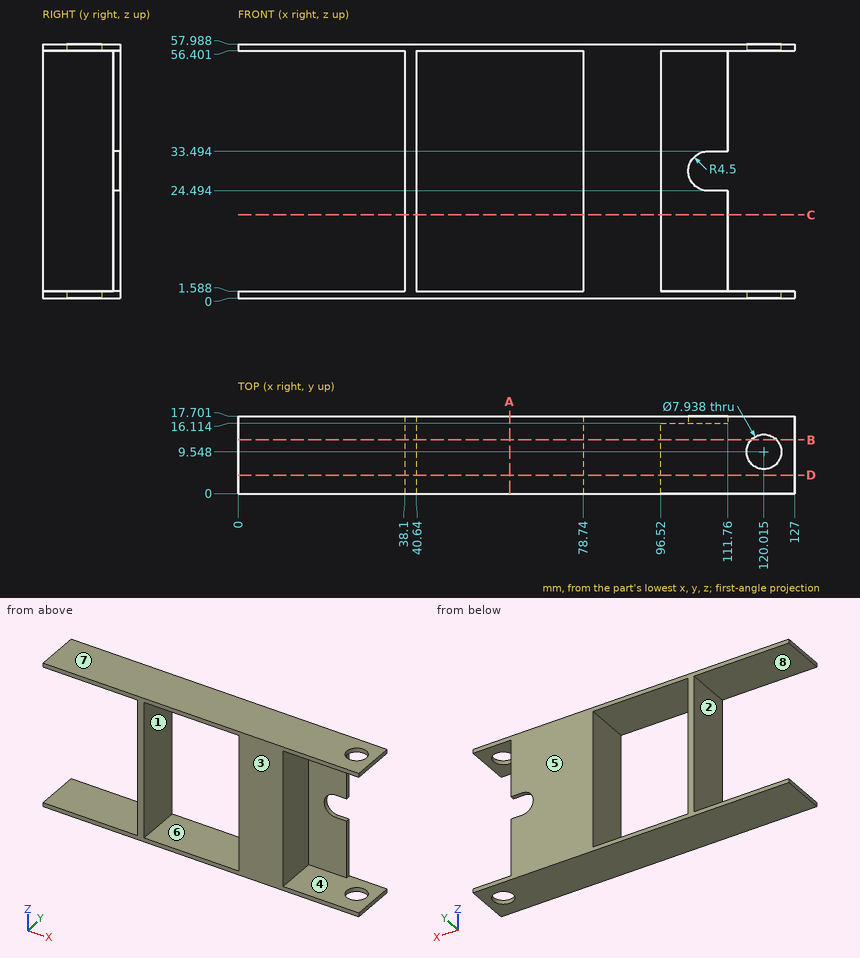
Here's the drawing with two shaded views (mm, measured from the low corner). I have some questions. A direction names the side the tool comes from. Give positions to 0.01 mm unless a question says otherwise; leave off trailing zeros. Order: outer loops, then holes, each group sorted by start corner. A loop starts at its lowest first (then second) coordinate and runs counter-clockwise, first axis right, second up. Notation, with made-up numbers: (-39, 63) - (12, 63) arc R27 ccw to (12, 98) - close; hole circle Ø5 at (0, 42). An arc over 180 degrees is marked (long way). Use a Markdown table: item, result. Add a question column.
Q1. On a 3-axis mill with a long thin cutter (end or side, diameter ignored), from which of +Z, -Z, +X, -X, +Y, -Y can I reach the whole of each face in a straight line? I mean the marked faces 4, 5, 6, 7 and 8. Say none if no direction works.
Q2. If we section it at B-B on y = 12.25: Write out the boundary of the cut face in (x, z).
Q3. Please list where these lines run through material, in increasing order: line 1 along X through (y, z) = (16.25, 51); line 2 along X through (y, z) = (7.5, 42); line 3 along Z through (x, y) = (7, 17).
Q4. If we section it at A-A on x = 62: Write out the boundary of the cut face in (y, z).
Q5. If we section it at C-C on z = 19: Write out the boundary of the cut face in (x, y).
Q6. If we section it at D-D on y = 4.25: Write out the boundary of the cut face in (x, z).
Q7. If we mould it in two halves opening along X, with no side actions, what happens to the marked faces 1, 2 and 3? For each: released by +X, released by -X, zero draft, split by the parting line, or undercut.
Q8. I'm going to push flat-ended pins straight in: pin 1 (6 mm diameter, centred on y = 5, z = 11.5, fed in from +X); pin 2 (1.5 mm diameter, centred on x = 99, z = 50.5, fed in from -Y); pin 3 (1.7 mm diameter, centred on y = 17, z = 42, fed in from +X). Where does each tip first touch, or does it pass through?
Answers follow:
| question | item | result |
|---|---|---|
| 1 | face 4 | +X, -Y |
| 1 | face 5 | +Z, -Z, +X, -X, +Y |
| 1 | face 6 | +Y, -Y |
| 1 | face 7 | +Z, +X, -X, +Y, -Y |
| 1 | face 8 | -X, +Y, -Y |
| 2 | outline | (0, 0) - (117.11, 0) - (117.11, 1.59) - (96.52, 1.59) - (96.52, 56.4) - (117.11, 56.4) - (117.11, 57.99) - (0, 57.99) - (0, 56.4) - (38.1, 56.4) - (38.1, 1.59) - (0, 1.59) - close; (122.92, 0) - (127, 0) - (127, 1.59) - (122.92, 1.59) - close; (122.92, 56.4) - (127, 56.4) - (127, 57.99) - (122.92, 57.99) - close; hole (40.64, 1.59) - (78.74, 1.59) - (78.74, 56.4) - (40.64, 56.4) - close |
| 3 | line 1 | x = 38.1 to 40.64, 78.74 to 111.76 |
| 3 | line 2 | x = 38.1 to 40.64, 78.74 to 96.52 |
| 3 | line 3 | z = 0 to 1.59, 56.4 to 57.99 |
| 4 | outline | (0, 0) - (17.7, 0) - (17.7, 1.59) - (0, 1.59) - close; (0, 56.4) - (17.7, 56.4) - (17.7, 57.99) - (0, 57.99) - close |
| 5 | outline | (38.1, 0) - (40.64, 0) - (40.64, 17.7) - (38.1, 17.7) - close; (78.74, 0) - (96.52, 0) - (96.52, 16.11) - (111.76, 16.11) - (111.76, 17.7) - (78.74, 17.7) - close |
| 6 | outline | (0, 0) - (127, 0) - (127, 1.59) - (96.52, 1.59) - (96.52, 56.4) - (127, 56.4) - (127, 57.99) - (0, 57.99) - (0, 56.4) - (38.1, 56.4) - (38.1, 1.59) - (0, 1.59) - close; hole (40.64, 1.59) - (78.74, 1.59) - (78.74, 56.4) - (40.64, 56.4) - close |
| 7 | face 1 | undercut |
| 7 | face 2 | released by -X |
| 7 | face 3 | zero draft |
| 8 | pin 1 | stops at x = 96.52 |
| 8 | pin 2 | stops at y = 16.11 |
| 8 | pin 3 | stops at x = 111.76 |
